Read the model definition and answer for the solid it produces. Units are mm, in the model's axes. A direction names the side the tool comes from. Give positions to 0.01 mm unless a question says otherwise; leave off trailing zeros. Order: outer loops, then holes, each group sorted by start corner. A loop starts at its lowest first (then second) coordinate and runs counter-clockwise, first axis right, second up. Notation, with made-up numbers: M 0.5,9 L 51.5,9 A16 cw 51.5,22 Z; hole C 44,-0.5 d3. An arc over 180 degrees is marked long. One line per item, written item: value.
from build123d import *

# Parameters (mm, degrees)
F1_W     = 500
F1_H     = 500
F2_DEPTH = 500
F3_W     = 385.679454
F3_H     = 350
F4_DEPTH = 350
F5_R     = 100


with BuildPart() as f2:
    # F1 (on face) → F2 (new body)
    with BuildSketch(Plane.XZ):
        with Locations((-250, 250)):
            Rectangle(F1_W, F1_H)
    extrude(amount=F2_DEPTH)

    # F3 (on face) → F4 (cut)
    with BuildSketch(Plane.XZ.offset(500)):
        with Locations((-192.839727, 325)):
            Rectangle(F3_W, F3_H)
    extrude(amount=-F4_DEPTH, mode=Mode.SUBTRACT)

    # F5
    f5_edges = [f2.edges().sort_by_distance(p)[0] for p in [
        (0, -500, 75),
    ]]
    fillet(f5_edges, radius=F5_R)


solid = f2.part
1) Find section B-B, the plane z = 419. Write down the section's boundary in (x, y), plus the area to 3 significant figures.
Reported:
outline: M -500,-500 L -385.68,-500 L -385.68,-150 L 0,-150 L 0,0 L -500,0 Z
area: 115,000 mm^2
2) Find section A-A, the plane x = -164.5. Write down the section's boundary in (y, z), plus the area to 4 significant figures.
Reported:
outline: M -500,0 L 0,0 L 0,500 L -150,500 L -150,150 L -500,150 Z
area: 127,500 mm^2
3) Which of the six approach directions +Z, -Z, +X, -X, +Y, -Y give full straight-line access (tool end or side, diameter ignored) to faces 1 (the face through (-385.679, -327, 323)), 2 (the face through (-253, 0, 254))?
Reported:
face 1: +Z, +X, -Y
face 2: +Z, -Z, +X, -X, +Y
4) Consider probe 1 along X at (y, z) = (-364.5, 153); probe 2 along Y at (x, z) = (-68, 223.5); probe 3 along Z at (x, y) = (-89, -470). Determine where each line is inside the solid, lowest interval first.
Reported:
probe 1: x = -500 to -385.68
probe 2: y = -150 to 0
probe 3: z = 0 to 150
5) This flat-tipped pin is pushed along its axis until it touches: pin 1 Ø4 at (y, z) = (-232.5, 418.5) entering from +X. Where does it stop, or does it pass through?
Reported:
pin 1: stops at x = -385.68
